Geometry check sheet. Reference: the model listing, model coordinates, mm. A direction names the side the tool comes from. Round coordinates to 2 decimals unless told otherwise and drop trailing zeros. Order: outer loops, then holes, each group sorted by start corner. A loop starts at its lowest first (then second) coordinate and runs counter-clockwise, first axis right, second up.
(1) Sectioned sample at A-A (y = 1). Record the boundary of the cut face in (x, z) (3 decimals), plus the area to 3 significant figures.
(2) Go/stop test with flat-tipped pins: pin 1 (7.5 mm diameter, centred on x = 36.32, z = 0, fed in from -Y); pin 2 (5.5 mm diameter, centred on y = 0.5, z = 33.5, fed in from +X); pin 3 (10 mm diameter, centred on y = -6.5, z = 23, fed in from -X); pin 4 (8 mm diameter, centred on y = -2.5, z = 27.5, fed in from -X). Record where each tip stops, or that it passes through.
(3) Sectioned sample at B-B (x = 36.5). Record the boundary of the cut face in (y, z).
(4) Material ranges on line 1 along X through (y, z) = (-4.5, 26.5); line 2 along Z through (x, y) = (28.25, -6.5); line 3 along Z through (x, y) = (32.75, -7.5), recorded low to high.
(5) Release check for a two-part mould opening along Z. For faces 1 (the face through (38.207, -0.07, -1.445)), 2 (the face through (36.2, -0.1, -4.3)), 3 (the face through (34, -5, 1)) record: +Z half, -Z half, draft (parallel to the pull), parting line (faces both ways), or undercut.
(6) Set-up check for faces 4 (the face through (24, 0, 30.636)), 5 (the face through (30.869, 0, 32)), 6 (the face through (36, 9, 4.302)): record each of +Z, -Z, +X, -X, +Y, -Y from which the full face is reachable in a straight line by a thin tool's end or side.
(7) Sectioned sample at C-C (y = 6.5). Record the boundary of the cut face in (x, z) (3 decimals), plus the area to 3 significant figures.
(8) Sectioned sample at D-D (z = 23.5). Record the boundary of the cut face in (x, y), plus the area to 3 significant figures.
from build123d import *

# Parameters (mm, degrees)
F1_DEPTH = 5
F2_DEPTH = 12.5
F4_DEPTH = 25


with BuildPart() as f1:
    # F0 (on Front) → F1 (new body, symmetric)
    with BuildSketch(Plane.XZ):
        with BuildLine():
            ThreePointArc((40.396538, 4.302366), (35.393921, 19.941439), (24.609375, 32.322891))
            Line((24.609375, 32.322891), (24.609375, 20.486002))
            ThreePointArc((24.609375, 20.486002), (29.308809, 12.895398), (31.729911, 4.302366))
            Line((31.729911, 4.302366), (36.322634, 4.302366))
            Line((36.322634, 4.302366), (40.396538, 4.302366))
        make_face()
        with BuildLine():
            ThreePointArc((32.020269, 0), (36.322634, -4.302366), (40.625, 0))
            Line((40.625, 0), (38.697634, 0))
            ThreePointArc((38.697634, 0), (36.322634, -2.375), (33.947634, 0))
            Line((33.947634, 0), (32.020269, 0))
        make_face()
        with BuildLine():
            Line((38.697634, 0), (40.625, 0))
            ThreePointArc((40.625, 0), (39.364866, 3.042232), (36.322634, 4.302366))
            ThreePointArc((36.322634, 4.302366), (33.280402, 3.042232), (32.020269, 0))
            Line((32.020269, 0), (33.947634, 0))
            ThreePointArc((33.947634, 0), (36.322634, 2.375), (38.697634, 0))
        make_face()
        with BuildLine():
            ThreePointArc((32.020269, 0), (33.280402, 3.042232), (36.322634, 4.302366))
            Line((36.322634, 4.302366), (31.729911, 4.302366))
            ThreePointArc((31.729911, 4.302366), (31.947597, 2.156076), (32.020269, 0))
        make_face()
        with BuildLine():
            ThreePointArc((36.322634, 4.302366), (39.364866, 3.042232), (40.625, 0))
            ThreePointArc((40.625, 0), (40.567844, 2.154214), (40.396538, 4.302366))
            Line((40.396538, 4.302366), (36.322634, 4.302366))
        make_face()
    extrude(amount=F1_DEPTH, both=True)

    # F0 (on Front) → F2 (join, symmetric)
    with BuildSketch(Plane.XZ):
        with BuildLine():
            ThreePointArc((40.396538, 4.302366), (35.393921, 19.941439), (24.609375, 32.322891))
            Line((24.609375, 32.322891), (24.609375, 20.486002))
            ThreePointArc((24.609375, 20.486002), (29.308809, 12.895398), (31.729911, 4.302366))
            Line((31.729911, 4.302366), (36.322634, 4.302366))
            Line((36.322634, 4.302366), (40.396538, 4.302366))
        make_face()
    extrude(amount=F2_DEPTH, both=True)

    # F3 (on face) → F4 (join)
    with BuildSketch(Plane.XZ.offset(12.5)):
        Polygon((24.609375, 30.636002), (24.609375, 20.486002), (30.868572, 20.486002), (30.868572, 37.486002), (24.609375, 37.486002), align=None)
        with BuildLine():
            Line((23.309375, 30.636002), (24.609375, 30.636002))
            Line((24.609375, 30.636002), (24.609375, 37.486002))
            Line((24.609375, 37.486002), (21.065177, 31.227315))
            ThreePointArc((21.065177, 31.227315), (22.415122, 31.796397), (23.309375, 30.636002))
        make_face()
        with BuildLine():
            ThreePointArc((21.065177, 31.227315), (21.803628, 29.475606), (23.309375, 30.636002))
            ThreePointArc((23.309375, 30.636002), (22.415122, 31.796397), (21.065177, 31.227315))
        make_face()
    extrude(amount=-F4_DEPTH)


solid = f1.part
Answer below:
1. outline: (21.065, 31.227) arc R1.2 ccw (long way) to (23.309, 30.636) - (24.609, 30.636) - (24.609, 20.486) arc R32.02 cw to (31.73, 4.302) arc R32.02 cw to (32.02, 0) arc R4.302 ccw to (40.625, 0) arc R40.625 ccw to (40.397, 4.302) arc R40.625 ccw to (30.869, 26.411) - (30.869, 37.486) - (24.609, 37.486) - close; hole circle Ø4.75 at (36.323, 0)
1. area: 334 mm2
2. pin 1: stops at y = -5
2. pin 2: stops at x = 30.87
2. pin 3: stops at x = 24.61
2. pin 4: stops at x = 20.91
3. outline: (-12.5, 4.3) - (-5, 4.3) - (-5, 2.37) - (5, 2.37) - (5, 4.3) - (12.5, 4.3) - (12.5, 17.84) - (-12.5, 17.84) - close; (-5, -4.3) - (5, -4.3) - (5, -2.37) - (-5, -2.37) - close
4. line 1: x = 24.61 to 30.87
4. line 2: z = 15.07 to 37.49
4. line 3: z = 4.3 to 24.04
5. face 1: undercut
5. face 2: -Z half
5. face 3: draft
6. face 4: -Z, +Y, -Y
6. face 5: +Z, +X, +Y, -Y
6. face 6: -Z, +X, -X, +Y
7. outline: (21.065, 31.227) arc R1.2 ccw (long way) to (23.309, 30.636) - (24.609, 30.636) - (24.609, 20.486) arc R32.02 cw to (31.73, 4.302) - (40.397, 4.302) arc R40.625 ccw to (30.869, 26.411) - (30.869, 37.486) - (24.609, 37.486) - close
7. area: 286 mm2
8. outline: (24.61, -12.5) - (33.14, -12.5) - (33.14, 12.5) - (24.61, 12.5) - close
8. area: 213 mm2
